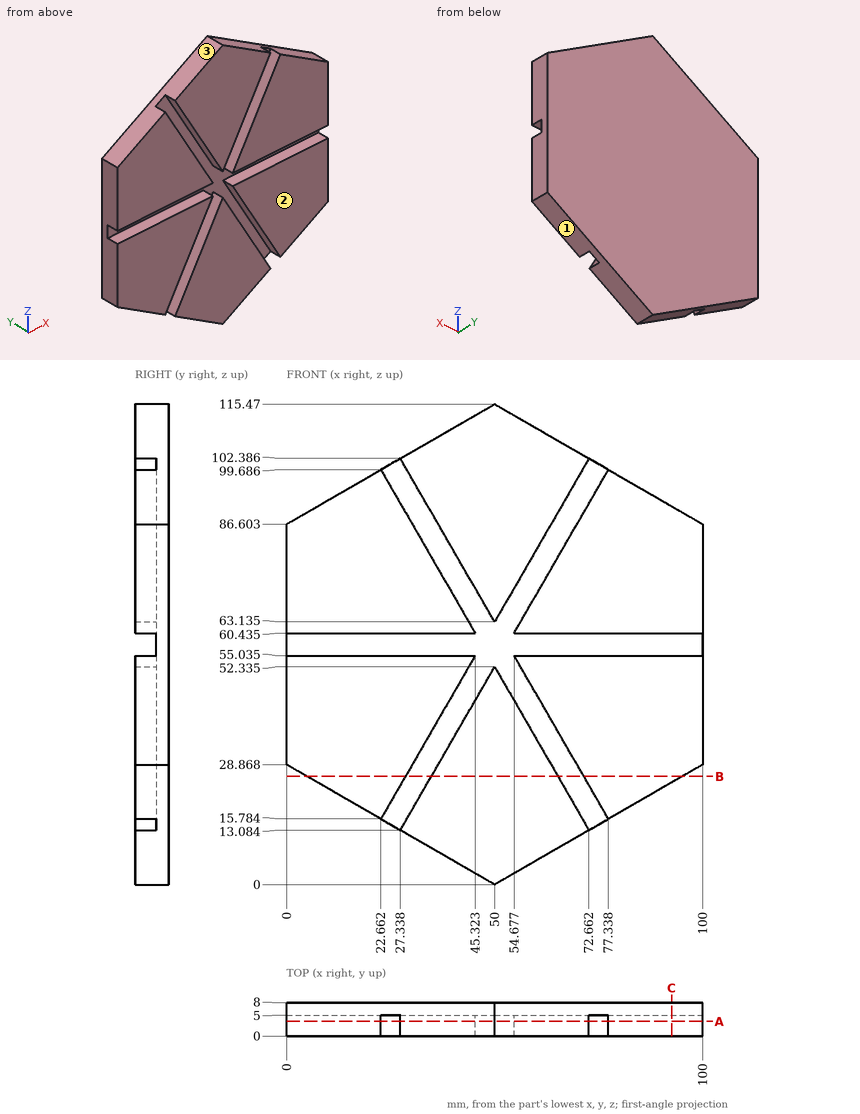
Job drawing, mm, ordinate dimensions from the low corner. One solid piece. Give positions to 0.01 mm unless a question says otherwise; leave off trailing zeros. Order: outer loops, then holes, each group sorted by start corner. A loop starts at its lowest first (then second) coordinate and runs counter-clockwise, first axis right, second up. Notation, with made-up numbers: M -15.5,-6 L 8.5,-6 A12 ccw 8.5,14 Z; hole C 71,-0.5 d9. An arc over 180 degrees is marked long. Put each result on its own line as item: value. Start each with the question number.
(1) Pull direction X, two halves, no side cores. Call the marked faces 1, 2 and 3: released by +X, released by -X, zero draft, split by the parting line, or undercut.
(2) Band-saw the part on A-A on y = 3.5. Give the cut face in (x, z) (1 decimal), then the cut area to 3 significant figures.
(3) Band-saw the part on C-C on x = 92.5. Give the cut face in (y, z) (1 decimal).
(4) Pin check, flat tips, straight feed: pin 1 Ø2.5 at (x, y) = (69, 2.5) entering from -Z; pin 2 Ø4 at (x, y) = (31, 2) entering from +Z (1 decimal); pin 3 Ø3 at (x, y) = (28.5, 6) entering from +Z. Stop position of each tip, or through.
(5) Drill centre lines: L1, parallel to Z at x = 69, y = 4 (1 decimal); L2, parallel to X at y = 2, z = 21 (1 decimal); L3, parallel to Z at x = 59.5, y = 1 (1 decimal). Where is each one in solid material? Low to high. Write a range as [from, to].
(6) Band-saw the part on B-B on z = 26. Give the cut face in (x, y) (1 decimal).
Results below:
1. face 1: released by +X
1. face 2: zero draft
1. face 3: released by -X
2. outline: M 0,28.9 L 22.7,15.8 L 45.3,55 L 0,55 Z; M 0,60.4 L 45.3,60.4 L 22.7,99.7 L 0,86.6 Z; M 27.3,13.1 L 50,0 L 72.7,13.1 L 50,52.3 Z; M 27.3,102.4 L 50,63.1 L 72.7,102.4 L 50,115.5 Z; M 54.7,55 L 77.3,15.8 L 100,28.9 L 100,55 Z; M 54.7,60.4 L 100,60.4 L 100,86.6 L 77.3,99.7 Z
2. area: 7,120 mm2
3. outline: M 0,24.5 L 8,24.5 L 8,90.9 L 0,90.9 L 0,60.4 L 5,60.4 L 5,55 L 0,55 Z
4. pin 1: stops at z = 10.25
4. pin 2: stops at z = 105.7
4. pin 3: stops at z = 103.92
5. L1: z = [11, 19.4], [30.2, 55], [60.4, 85.2], [96, 104.5]
5. L2: x = [13.6, 25.7], [31.9, 68.1], [74.3, 86.4]
5. L3: z = [5.5, 35.9], [46.7, 55], [60.4, 68.8], [79.6, 110]
6. outline: M 5,0 L 28.6,0 L 28.6,5 L 34.8,5 L 34.8,0 L 65.2,0 L 65.2,5 L 71.4,5 L 71.4,0 L 95,0 L 95,8 L 5,8 Z
